from build123d import *

# Parameters (mm, degrees)
F1_DEPTH     = 9.79181
F2_T         = -2.5
F3_R         = 5
F4_T1_DEPTH  = 80
F4_T3_DEPTH  = 40
F4_T6_ANGLE  = 90
F4_T8_ANGLE  = 90
F4_T10_ANGLE = 90
F4_T12_ANGLE = 90
F5_R         = 7
F6_R         = 4.5
F7_DEPTH     = 130
F8_T         = -2.5
F12_DEPTH    = 6.2
F13_R        = 0.3
F14_R        = 0.3
F15_W        = 12
F15_H        = 4.35
F16_DEPTH    = 67.90149


# Not quite as in the source:
# - a fillet or chamfer that OpenCascade refuses, or shapes differently, is made with other operations: its cross-section is extruded or revolved along the edge and cut away or added


with BuildPart() as f1:
    # F0 (on Front) → F1 (new body)
    with BuildSketch(Plane.XZ):
        with BuildLine():
            Line((33.4467580169, 25.7645070341), (-46.5532419831, 25.7645070341))
            ThreePointArc((-46.5532419831, 25.7645070341), (-50.088775889, 24.30004094), (-51.5532419831, 20.7645070341))
            Line((-51.5532419831, 20.7645070341), (-51.5532419831, -19.2354929659))
            ThreePointArc((-51.5532419831, -19.2354929659), (-50.088775889, -22.7710268718), (-46.5532419831, -24.2354929659))
            Line((-46.5532419831, -24.2354929659), (33.4467580169, -24.2354929659))
            ThreePointArc((33.4467580169, -24.2354929659), (36.9822919229, -22.7710268718), (38.4467580169, -19.2354929659))
            Line((38.4467580169, -19.2354929659), (38.4467580169, 20.7645070341))
            ThreePointArc((38.4467580169, 20.7645070341), (36.9822919229, 24.30004094), (33.4467580169, 25.7645070341))
        make_face()
    extrude(amount=F1_DEPTH)

    # F2
    f2_openings = [f1.faces().sort_by_distance(p)[0] for p in [
        (-6.553242, -9.79181, 0.764507),
    ]]
    offset(amount=F2_T, openings=f2_openings)

    # F3
    f3_edges = [f1.edges().sort_by_distance(p)[0] for p in [
        (-6.553242, -2.5, 23.264507),
    ]]
    fillet(f3_edges, radius=F3_R)

    # F4: fillet of radius 5 on 1 edges, made by hand

    # F4_s2 → F4_t1 (cut)
    with BuildSketch(Plane.YZ.offset(-46.5532419831)):
        with BuildLine():
            ThreePointArc((-6.145905, 23.0776584685), (-8.7774388713, 24.8717434082), (-9.79181, 27.890809903))
            Line((-9.79181, 27.890809903), (-10.29181, 27.890809903))
            Line((-10.29181, 27.890809903), (-10.29181, 23.2645070341))
            Line((-10.29181, 23.2645070341), (-9.79181, 22.7645070341))
            ThreePointArc((-9.79181, 22.7645070341), (-7.5, 22.7645070341), (-6.2813145, 22.5963433251))
            Line((-6.2813145, 22.5963433251), (-6.145905, 23.0776584685))
        make_face()
        with BuildLine():
            ThreePointArc((-9.79181, -26.3617958348), (-8.7774388713, -23.34272934), (-6.145905, -21.5486444004))
            Line((-6.145905, -21.5486444004), (-6.2813145, -21.0673292569))
            ThreePointArc((-6.2813145, -21.0673292569), (-7.5, -21.2354929659), (-9.79181, -21.2354929659))
            Line((-9.79181, -21.2354929659), (-10.29181, -21.7354929659))
            Line((-10.29181, -21.7354929659), (-10.29181, -26.3617958348))
            Line((-10.29181, -26.3617958348), (-9.79181, -26.3617958348))
        make_face()
    extrude(amount=F4_T1_DEPTH, mode=Mode.SUBTRACT)

    # F4_s4 → F4_t3 (cut)
    with BuildSketch(Plane.XY.offset(-19.2354929659)):
        with BuildLine():
            ThreePointArc((-53.679544852, -9.79181), (-50.6604783572, -8.7774388713), (-48.8663934175, -6.145905))
            Line((-48.8663934175, -6.145905), (-48.3850782741, -6.2813145))
            ThreePointArc((-48.3850782741, -6.2813145), (-48.5532419831, -7.5), (-48.5532419831, -9.79181))
            Line((-48.5532419831, -9.79181), (-49.0532419831, -10.29181))
            Line((-49.0532419831, -10.29181), (-53.679544852, -10.29181))
            Line((-53.679544852, -10.29181), (-53.679544852, -9.79181))
        make_face()
        with BuildLine():
            ThreePointArc((40.5730608858, -9.79181), (37.5539943911, -8.7774388713), (35.7599094514, -6.145905))
            Line((35.7599094514, -6.145905), (35.278594308, -6.2813145))
            ThreePointArc((35.278594308, -6.2813145), (35.4467580169, -7.5), (35.4467580169, -9.79181))
            Line((35.4467580169, -9.79181), (35.9467580169, -10.29181))
            Line((35.9467580169, -10.29181), (40.5730608858, -10.29181))
            Line((40.5730608858, -10.29181), (40.5730608858, -9.79181))
        make_face()
    extrude(amount=F4_T3_DEPTH, mode=Mode.SUBTRACT)

    # F4_s5 → F4_t6 (revolve, cut)
    with BuildSketch(Plane.XY.offset(20.7645070341)):
        with BuildLine():
            ThreePointArc((35.9467580169, -4.79181), (37.411224111, -8.3273439059), (40.9467580169, -9.79181))
            Line((40.9467580169, -9.79181), (40.9467580169, -9.89181))
            Line((40.9467580169, -9.89181), (35.8467580169, -9.89181))
            Line((35.8467580169, -9.89181), (35.8467580169, -4.79181))
            Line((35.8467580169, -4.79181), (35.9467580169, -4.79181))
        make_face()
    revolve(axis=Axis((33.4467580169, -9.79181, 20.7645070341), (0, -1, 0)), revolution_arc=F4_T6_ANGLE, mode=Mode.SUBTRACT)

    # F4_s7 → F4_t8 (revolve, cut)
    with BuildSketch(Plane.YZ.offset(-46.5532419831)):
        with BuildLine():
            ThreePointArc((-9.79181, 28.2645070341), (-8.3273439059, 24.7289731282), (-4.79181, 23.2645070341))
            Line((-4.79181, 23.2645070341), (-4.79181, 23.1645070341))
            Line((-4.79181, 23.1645070341), (-9.89181, 23.1645070341))
            Line((-9.89181, 23.1645070341), (-9.89181, 28.2645070341))
            Line((-9.89181, 28.2645070341), (-9.79181, 28.2645070341))
        make_face()
    revolve(axis=Axis((-46.5532419831, -9.79181, 20.7645070341), (0, -1, 0)), revolution_arc=F4_T8_ANGLE, mode=Mode.SUBTRACT)

    # F4_s9 → F4_t10 (revolve, cut)
    with BuildSketch(Plane.XY.offset(-19.2354929659)):
        with BuildLine():
            ThreePointArc((-54.0532419831, -9.79181), (-50.5177080771, -8.3273439059), (-49.0532419831, -4.79181))
            Line((-49.0532419831, -4.79181), (-48.9532419831, -4.79181))
            Line((-48.9532419831, -4.79181), (-48.9532419831, -9.89181))
            Line((-48.9532419831, -9.89181), (-54.0532419831, -9.89181))
            Line((-54.0532419831, -9.89181), (-54.0532419831, -9.79181))
        make_face()
    revolve(axis=Axis((-46.5532419831, -9.79181, -19.2354929659), (0, -1, 0)), revolution_arc=F4_T10_ANGLE, mode=Mode.SUBTRACT)

    # F4_s11 → F4_t12 (revolve, cut)
    with BuildSketch(Plane.YZ.offset(33.4467580169)):
        with BuildLine():
            ThreePointArc((-9.79181, -26.7354929659), (-8.3273439059, -23.19995906), (-4.79181, -21.7354929659))
            Line((-4.79181, -21.7354929659), (-4.79181, -21.6354929659))
            Line((-4.79181, -21.6354929659), (-9.89181, -21.6354929659))
            Line((-9.89181, -21.6354929659), (-9.89181, -26.7354929659))
            Line((-9.89181, -26.7354929659), (-9.79181, -26.7354929659))
        make_face()
    revolve(axis=Axis((33.4467580169, -9.79181, -19.2354929659), (0, -1, 0)), revolution_arc=F4_T12_ANGLE, mode=Mode.SUBTRACT)

    # F5
    f5_edges = [f1.edges().sort_by_distance(p)[0] for p in [
        (-6.553242, 0, 25.764507),
    ]]
    fillet(f5_edges, radius=F5_R)


with BuildPart() as f7:
    # F6 (on Front) → F7 (new body)
    with BuildSketch(Plane.XZ):
        with Locations((-6.3970589777, 0)):
            Circle(F6_R)
    extrude(amount=-F7_DEPTH)

    # F8
    f8_openings = [f7.faces().sort_by_distance(p)[0] for p in [
        (-6.397059, 130, 0),
    ]]
    offset(amount=F8_T, openings=f8_openings)


with BuildPart() as f12:
    # F11 (on Front) → F12 (new body)
    with BuildSketch(Plane.XZ):
        with BuildLine():
            Line((-43.4241547674, 46.4492497861), (-55.8741547674, 46.4492497861))
            ThreePointArc((-55.8741547674, 46.4492497861), (-59.4096886733, 44.9847836921), (-60.8741547674, 41.4492497861))
            Line((-60.8741547674, 41.4492497861), (-60.8741547674, 11.5992497861))
            Line((-60.8741547674, 11.5992497861), (-58.6241547674, 11.5992497861))
            Line((-58.6241547674, 11.5992497861), (-58.6241547674, 13.1492497861))
            Line((-58.6241547674, 13.1492497861), (-59.6741547674, 13.1492497861))
            Line((-59.6741547674, 13.1492497861), (-59.6741547674, 19.5992497861))
            Line((-59.6741547674, 19.5992497861), (-58.7741547674, 19.5992497861))
            Line((-58.7741547674, 19.5992497861), (-58.7741547674, 21.0992497861))
            Line((-58.7741547674, 21.0992497861), (-59.6741547674, 21.0992497861))
            Line((-59.6741547674, 21.0992497861), (-59.6741547674, 33.2492497861))
            Line((-59.6741547674, 33.2492497861), (-58.7741547674, 33.2492497861))
            Line((-58.7741547674, 33.2492497861), (-58.7741547674, 34.7492497861))
            Line((-58.7741547674, 34.7492497861), (-59.6741547674, 34.7492497861))
            Line((-59.6741547674, 34.7492497861), (-59.6741547674, 41.4492497861))
            ThreePointArc((-59.6741547674, 41.4492497861), (-58.5611605359, 44.1362555546), (-55.8741547674, 45.2492497861))
            Line((-55.8741547674, 45.2492497861), (-43.4241547674, 45.2492497861))
            ThreePointArc((-43.4241547674, 45.2492497861), (-40.7371489989, 44.1362555546), (-39.6241547674, 41.4492497861))
            Line((-39.6241547674, 41.4492497861), (-39.6241547674, 34.7492497861))
            Line((-39.6241547674, 34.7492497861), (-40.5241547674, 34.7492497861))
            Line((-40.5241547674, 34.7492497861), (-40.5241547674, 33.2492497861))
            Line((-40.5241547674, 33.2492497861), (-39.6241547674, 33.2492497861))
            Line((-39.6241547674, 33.2492497861), (-39.6241547674, 21.0992497861))
            Line((-39.6241547674, 21.0992497861), (-40.5241547674, 21.0992497861))
            Line((-40.5241547674, 21.0992497861), (-40.5241547674, 19.5992497861))
            Line((-40.5241547674, 19.5992497861), (-39.6241547674, 19.5992497861))
            Line((-39.6241547674, 19.5992497861), (-39.6241547674, 13.1492497861))
            Line((-39.6241547674, 13.1492497861), (-40.6741547674, 13.1492497861))
            Line((-40.6741547674, 13.1492497861), (-40.6741547674, 11.5992497861))
            Line((-40.6741547674, 11.5992497861), (-38.4241547674, 11.5992497861))
            Line((-38.4241547674, 11.5992497861), (-38.4241547674, 41.4492497861))
            ThreePointArc((-38.4241547674, 41.4492497861), (-39.8886208615, 44.9847836921), (-43.4241547674, 46.4492497861))
        make_face()
    extrude(amount=F12_DEPTH)

    # F13
    f13_edges = [f12.edges().sort_by_distance(p)[0] for p in [
        (-59.674155, -3.1, 13.14925),
    ]]
    fillet(f13_edges, radius=F13_R)

    # F14
    f14_edges = [f12.edges().sort_by_distance(p)[0] for p in [
        (-39.624155, -3.1, 13.14925),
    ]]
    fillet(f14_edges, radius=F14_R)

    # F15 (on Top) → F16 (cut)
    with BuildSketch(Plane.XY):
        with Locations((-49.6491547674, -3.1)):
            Rectangle(F15_W, F15_H)
    extrude(amount=F16_DEPTH, mode=Mode.SUBTRACT)


solid = f12.part
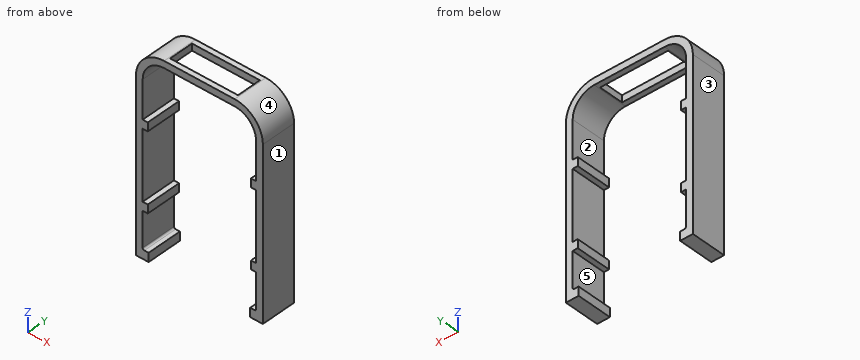
Part model, mm, in its own coordinate system. Face numbers are marked on the shaded views. A direction names the side the tool comes from. Round coordinates to 2 decimals unless told otherwise and drop trailing zeros. Order: outer loops, then holes, each group sorted by start corner. A loop starts at its lowest first (then second) coordinate and runs counter-clockwise, first axis right, second up. Notation, with made-up numbers: (48.5, 71) -> (88.5, 71) arc R22 ccw to (88.5, 79) -> close; hole circle Ø11 at (-8, -10.75). An arc over 180 degrees is marked (long way). Put each result on its own line as item: value.
Q1. Tool access for the marked faces 4 and 5: list every direction of +Z, -Z, +X, -X, +Y, -Y with a clear straight run to the whole face (end or side of a thin tool).
From the geometry:
face 4: +Z, +X, +Y, -Y
face 5: +Y, -Y
Q2. Wall check: line 1 (X direction, y = -4, z = 19); line 2 (Z direction, x = -40, y = -1.75); line 3 (Z direction, x = -43.5, y = -3.25). Give the ranges that are in metal, low to high. Write a range as [from, to].
From the geometry:
line 1: x = [-60.87, -59.67], [-39.62, -38.42]
line 2: z = [11.6, 13.15], [19.6, 21.1], [33.25, 34.75], [43.1, 45.09]
line 3: z = [45.25, 46.45]
Q3. Band-saw the part on B-B (z = 17). Give the cut face in (x, y), and give its area (3 significant figures).
From the geometry:
outline: (-60.87, -6.2) -> (-59.67, -6.2) -> (-59.67, 0) -> (-60.87, 0) -> close; (-39.62, -6.2) -> (-38.42, -6.2) -> (-38.42, 0) -> (-39.62, 0) -> close
area: 14.9 mm2
Q4. Band-saw the part on A-A (x = -50.25). Give the cut face in (y, z) (3 decimals).
From the geometry:
outline: (-6.2, 45.249) -> (-5.275, 45.249) -> (-5.275, 46.449) -> (-6.2, 46.449) -> close; (-0.925, 45.249) -> (0, 45.249) -> (0, 46.449) -> (-0.925, 46.449) -> close
Q5. Band-saw the part on C-C (x = -42.5). Give the cut face in (y, z).
From the geometry:
outline: (-6.2, 45.14) -> (0, 45.14) -> (0, 46.36) -> (-6.2, 46.36) -> close
Q6. Band-saw the part on D-D (x = -56.5). Give the cut face in (y, z), and give its area (3 significant figures).
From the geometry:
outline: (-6.2, 45.2) -> (0, 45.2) -> (0, 46.41) -> (-6.2, 46.41) -> close
area: 7.52 mm2
Q7. Pin check, flat tips, straight feed: pin 1 Ø0.8 at (x, y) = (-59, -3) entering from +Z; pin 2 Ø1 at (y, z) = (-3, 46) entering from -X. Stop position of each tip, or through.
From the geometry:
pin 1: stops at z = 45.64
pin 2: stops at x = -58.81
Q8. Pull direction X, two halves, no side cores. Call the marked faces 1, 2 and 3: pulls with the +X half, pulls with the -X half, needs draft (parallel to the pull), parting line crosses it, or undercut.
From the geometry:
face 1: pulls with the +X half
face 2: undercut
face 3: pulls with the -X half
